from build123d import *
from OCP.BRepFilletAPI import BRepFilletAPI_MakeChamfer

# Parameters (mm, degrees)
BOSS_EXTRU_1_DEPTH      = 50
CHANFREIN1_SIZE         = 20
ENL_V_MAT_EXTRU_1_DEPTH = 10
CHANFREIN2_SIZE         = 10
CHANFREIN2_SIZE_2       = 17.320508076
CHANFREIN3_SIZE         = 5
ENL_V_MAT_EXTRU_2_DEPTH = 30
ESQUISSE4_W             = 311.726027397
ESQUISSE4_H             = 51.931996983
ENL_V_MAT_EXTRU_3_DEPTH = 681.504586336


# Some blends are built 0.0001 mm under size
with BuildPart() as part:
    # Esquisse1 → Boss.-Extru.1 (new body)
    with BuildSketch(Plane.XY):
        Polygon((0, 0), (219.726027397, 0), (269.726027397, 50), (269.726027397, 176.794919243), (169.726027397, 350), (8, 350), (-42, 300), (-42, 72.746133918), align=None)
    extrude(amount=BOSS_EXTRU_1_DEPTH)

    # Chanfrein1
    chanfrein1_edges = [part.edges().sort_by_distance(p)[0] for p in [
        (244.726027397, 25, 50),
        (269.726027397, 113.397459622, 50),
        (219.726027397, 263.397459622, 50),
        (88.863013699, 350, 50),
        (-17, 325, 50),
        (-42, 186.373066959, 50),
        (-21, 36.373066959, 50),
        (109.863013699, 0, 50),
    ]]
    chamfer(chanfrein1_edges, length=CHANFREIN1_SIZE)

    # Esquisse2 → Enlèv. mat.-Extru.1 (cut)
    with BuildSketch(Plane.XY.offset(50)):
        Polygon((28.710678119, 300), (219.726027397, 70.710678119), (219.726027397, 163.397459622), (140.858513938, 300), align=None)
        Polygon((199.015349279, 50), (8, 279.289321881), (8, 86.143593539), (28.867513459, 50), align=None)
    extrude(amount=-ENL_V_MAT_EXTRU_1_DEPTH, mode=Mode.SUBTRACT)

    # Chanfrein2
    chanfrein2_edges_1 = [part.edges().sort_by_distance(p)[0] for p in [
        (219.726027397, 117.05406887, 40),
    ]]
    chanfrein2_side_1 = [part.faces().sort_by_distance(p)[0] for p in [
        (219.726027397, 117.05406887, 40.2),
    ]]
    chanfrein2_edges_2 = [part.edges().sort_by_distance(p)[0] for p in [
        (180.292270668, 231.698729811, 40),
    ]]
    chanfrein2_side_2 = [part.faces().sort_by_distance(p)[0] for p in [
        (180.292270668, 231.698729811, 40.2),
    ]]
    chanfrein2_edges_3 = [part.edges().sort_by_distance(p)[0] for p in [
        (84.784596028, 300, 40),
    ]]
    chanfrein2_side_3 = [part.faces().sort_by_distance(p)[0] for p in [
        (84.784596028, 300, 40.2),
    ]]
    chanfrein2_edges_4 = [part.edges().sort_by_distance(p)[0] for p in [
        (113.941431369, 50, 40),
    ]]
    chanfrein2_side_4 = [part.faces().sort_by_distance(p)[0] for p in [
        (113.941431369, 50, 40.2),
    ]]
    chanfrein2_edges_5 = [part.edges().sort_by_distance(p)[0] for p in [
        (18.43375673, 68.07179677, 40),
    ]]
    chanfrein2_side_5 = [part.faces().sort_by_distance(p)[0] for p in [
        (18.43375673, 68.07179677, 40.2),
    ]]
    chanfrein2_edges_6 = [part.edges().sort_by_distance(p)[0] for p in [
        (8, 182.71645771, 40),
    ]]
    chanfrein2_side_6 = [part.faces().sort_by_distance(p)[0] for p in [
        (8, 182.71645771, 40.2),
    ]]
    chanfrein2 = BRepFilletAPI_MakeChamfer(part.part.solid().wrapped)
    for e in chanfrein2_edges_1:
        chanfrein2.Add(CHANFREIN2_SIZE - 0.0001, CHANFREIN2_SIZE_2 - 0.0001, e.wrapped, chanfrein2_side_1[0].wrapped)
    for e in chanfrein2_edges_2:
        chanfrein2.Add(CHANFREIN2_SIZE - 0.0001, CHANFREIN2_SIZE_2 - 0.0001, e.wrapped, chanfrein2_side_2[0].wrapped)
    for e in chanfrein2_edges_3:
        chanfrein2.Add(CHANFREIN2_SIZE - 0.0001, CHANFREIN2_SIZE_2 - 0.0001, e.wrapped, chanfrein2_side_3[0].wrapped)
    for e in chanfrein2_edges_4:
        chanfrein2.Add(CHANFREIN2_SIZE - 0.0001, CHANFREIN2_SIZE_2 - 0.0001, e.wrapped, chanfrein2_side_4[0].wrapped)
    for e in chanfrein2_edges_5:
        chanfrein2.Add(CHANFREIN2_SIZE - 0.0001, CHANFREIN2_SIZE_2 - 0.0001, e.wrapped, chanfrein2_side_5[0].wrapped)
    for e in chanfrein2_edges_6:
        chanfrein2.Add(CHANFREIN2_SIZE - 0.0001, CHANFREIN2_SIZE_2 - 0.0001, e.wrapped, chanfrein2_side_6[0].wrapped)
    add(Compound.cast(chanfrein2.Shape()), mode=Mode.REPLACE)  # a hair under: the kernel refuses the full size

    # Chanfrein3
    # the kernel refuses this chamfer: 5 mm, written as the material it takes off along each edge
    with BuildSketch(Plane(origin=(20.480424013, 309.879359904, 50), x_dir=(-0.768028153682994, -0.6398255480361086, 0.02749587661058626), z_dir=(0.6400675467511631, -0.7683186419682577, 0))) as chanfrein3_piece_1_section:
        Polygon((CHANFREIN3_SIZE * 0.999621916911, CHANFREIN3_SIZE * 0.0274958766106), (-CHANFREIN3_SIZE * 0.0274958766106, CHANFREIN3_SIZE * 0.999621916911), (0, 0), align=None)
    chanfrein3_piece_1 = extrude(amount=324.14681629, mode=Mode.PRIVATE)
    chanfrein3_piece_1 = split(chanfrein3_piece_1, bisect_by=Plane(origin=(122.894695162, 300, 48.383637618), z_dir=(0, -1, 0)), keep=Keep.TOP, mode=Mode.PRIVATE)
    chanfrein3_piece_1 = split(chanfrein3_piece_1, bisect_by=Plane(origin=(122.894695162, 212.546373523, -0.491261384), z_dir=(0, -0.4999984150451088, 0.8660263188566379)), keep=Keep.TOP, mode=Mode.PRIVATE)
    chanfrein3_piece_1 = split(chanfrein3_piece_1, bisect_by=Plane(origin=(219.726027397, 184.328556692, 48.383637618), z_dir=(-1, 0, 0)), keep=Keep.TOP, mode=Mode.PRIVATE)
    chanfrein3_piece_1 = split(chanfrein3_piece_1, bisect_by=Plane(origin=(146.402514085, 184.328556692, 7.666728775), z_dir=(-0.49999841504510817, 0, 0.8660263188566384)), keep=Keep.TOP, mode=Mode.PRIVATE)
    add(chanfrein3_piece_1, mode=Mode.SUBTRACT)
    with BuildSketch(Plane(origin=(207.245603384, 40.120640096, 50), x_dir=(-0.02112559457717319, -0.017599218287911274, -0.9996219169112968), z_dir=(-0.6400675467511632, 0.7683186419682577, 0))) as chanfrein3_piece_2_section:
        Polygon((CHANFREIN3_SIZE * 0.999621916911, -CHANFREIN3_SIZE * 0.0274958766106), (-CHANFREIN3_SIZE * 0.0274958766106, -CHANFREIN3_SIZE * 0.999621916911), (0, 0), align=None)
    chanfrein3_piece_2 = extrude(amount=324.14681629, mode=Mode.PRIVATE)
    chanfrein3_piece_2 = split(chanfrein3_piece_2, bisect_by=Plane(origin=(104.831332235, 50, 48.383637618), z_dir=(0, 1, 0)), keep=Keep.TOP, mode=Mode.PRIVATE)
    chanfrein3_piece_2 = split(chanfrein3_piece_2, bisect_by=Plane(origin=(104.831332235, 137.453626477, -0.491261384), z_dir=(0, 0.4999984150451082, 0.8660263188566383)), keep=Keep.TOP, mode=Mode.PRIVATE)
    chanfrein3_piece_2 = split(chanfrein3_piece_2, bisect_by=Plane(origin=(8, 165.671443308, 48.383637618), z_dir=(1, 0, 0)), keep=Keep.TOP, mode=Mode.PRIVATE)
    chanfrein3_piece_2 = split(chanfrein3_piece_2, bisect_by=Plane(origin=(81.323513312, 165.671443308, 7.666728775), z_dir=(0.49999841504510834, 0, 0.8660263188566383)), keep=Keep.TOP, mode=Mode.PRIVATE)
    add(chanfrein3_piece_2, mode=Mode.SUBTRACT)

    # Esquisse3 → Enlèv. mat.-Extru.2 (cut)
    with BuildSketch(Plane(origin=(0, 0, 0), x_dir=(-1, 0, 0), z_dir=(0, 0, -1))):
        Polygon((-5.773502692, 10), (32, 75.425625842), (32, 295.857864376), (-12.142135624, 340), (-163.952524705, 340), (-259.726027397, 174.115427319), (-259.726027397, 54.142135624), (-215.583891774, 10), align=None)
    extrude(amount=-ENL_V_MAT_EXTRU_2_DEPTH, mode=Mode.SUBTRACT)

    # Symétrie1: part across plane


with BuildPart() as part_1:
    add(part.part)
    add(part.part.mirror(Plane(origin=(269.726027397, 50, 50), x_dir=(0, 0, 1), z_dir=(-1, 0, 0))))

    # Esquisse4 → Enlèv. mat.-Extru.3 (cut, through all)
    with BuildSketch(Plane(origin=(0, 350, 0), x_dir=(1, 0, 0), z_dir=(0, 1, 0))):
        with Locations((113.863013698, -25.965998492)):
            Rectangle(ESQUISSE4_W, ESQUISSE4_H)
    extrude(amount=-ENL_V_MAT_EXTRU_3_DEPTH, mode=Mode.SUBTRACT)


solid = part_1.part
Can you work these out from the model? Positions are in its coordinate system, mm. A direction names the side the tool comes from. Give positions to 0.01 mm unless a question says otherwise; leave off trailing zeros. Loops run counter-clockwise (first coordinate to the right, second up) from the corner with the lowest first, then second, coordinate; pieces in that order, holes last. Notation, with made-up numbers: (-36.5, 25) - (9.5, 25) arc R26 cw to (9.5, 41) - close; hole circle Ø9 at (75.25, 20.25). An arc over 180 degrees is marked (long way). Answer as a JSON object with one key per item and string values.
Q1. If we mould it in two halves opening along X, with no side actions, what happens to faces 4 (the flat face through (366.21, 226.35, 44.93)), 5 (the flat face through (513.56, 72.72, 44.93)), 6 (the flat face through (431, 0, 15)), 7 (the flat face through (269.726, 114, 15))? For each: pulls with the +X half, pulls with the -X half, needs draft (parallel to the pull), parting line crosses it, or undercut.
Geometry says:
{"face 4": "undercut", "face 5": "undercut", "face 6": "needs draft", "face 7": "pulls with the -X half"}
Q2. Will these pins go through, and if not, where does the flat tip stop? P1, Ø10, axis at y = 87.5, z = 37, coming from the -X side; P2, Ø3, axis at x = 333, y = 152.5, coming from the +Z side; P3, Ø3, axis at y = 256.5, z = 8.5, coming from the -X side.
Geometry says:
{"P1": "x = 271.73", "P2": "z = 43.2", "P3": "x = 314.88"}
Q3. Imagine slicing it at D-D on x = 547. Write out the boundary of the cut face in (y, z).
Geometry says:
{"outline": "(13.07, 0) - (33.07, 0) - (33.07, 30) - (320.31, 30) - (320.31, 0) - (334.45, 0) - (334.45, 30) - (306.17, 50) - (53.07, 50) - (13.07, 30) - close"}
Q4. Which directions (+Z, -Z, +X, -X, +Y, -Y) give clear straight access to the entire face, cutting with the end or side of a thin tool? Please do faces 1 (the flat face through (434, 162.31, 42.54)), 2 (the flat face through (576, 163, 0)), 3 (the flat face through (328.283, 258.219, 14.79)).
Geometry says:
{"face 1": "+Z", "face 2": "-Z, +X, -X, +Y, -Y", "face 3": "-Z"}
Q5. Imagine slicing it at A-A on z = 6. Write out the boundary of the cut face in (x, y), plus the area to 3 significant figures.
Geometry says:
{"outline": "(269.73, 50) - (319.73, 0) - (539.45, 0) - (581.45, 72.75) - (581.45, 300) - (531.45, 350) - (369.73, 350) - (269.73, 176.79) - close; hole (279.73, 54.14) - (323.87, 10) - (533.68, 10) - (571.45, 75.43) - (571.45, 295.86) - (527.31, 340) - (375.5, 340) - (279.73, 174.12) - close", "area": "11,300 mm²"}
Q6. If I drill on L1, parallel to Y at x = 449, z = 8.5; L2, parallel to X at y = 129, z = 23.5; L3, parallel to Z at x = 411, y = 278.5, over which ranges is the centre line in solid material (lowest first)?
Geometry says:
{"L1": "0 to 10, 340 to 350", "L2": "269.73 to 279.73, 571.45 to 581.45", "L3": "30 to 40"}
